from build123d import *

# Parameters (mm, degrees)
SKETCH1_R           = 1.95
SKETCH1_R_2         = 1.1
SKETCH1_R_3         = 1.7
SKETCH1_W           = 20
SKETCH1_H           = 3
BOSS_EXTRUDE2_DEPTH = 2


with BuildPart() as part:
    # Sketch1 → Boss-Extrude2 (new body)
    with BuildSketch(Plane.XY):
        with BuildLine():
            Line((-132.281780802, 145), (45.918219198, 145))
            ThreePointArc((45.918219198, 145), (47.332432761, 144.414213562), (47.918219198, 143))
            Line((47.918219198, 143), (47.918219198, 137))
            ThreePointArc((47.918219198, 137), (47.332432761, 135.585786438), (45.918219198, 135))
            Line((45.918219198, 135), (30.918219198, 135))
            ThreePointArc((30.918219198, 135), (30.211112417, 134.707106781), (29.918219198, 134))
            Line((29.918219198, 134), (29.918219198, 11))
            ThreePointArc((29.918219198, 11), (30.211112417, 10.292893219), (30.918219198, 10))
            Line((30.918219198, 10), (45.918219198, 10))
            ThreePointArc((45.918219198, 10), (47.332432761, 9.414213562), (47.918219198, 8))
            Line((47.918219198, 8), (47.918219198, 2))
            ThreePointArc((47.918219198, 2), (47.332432761, 0.585786438), (45.918219198, 0))
            Line((45.918219198, 0), (29.918219198, 0))
            Line((29.918219198, 0), (29.918219198, -44.1))
            ThreePointArc((29.918219198, -44.1), (29.62532598, -44.807106781), (28.918219198, -45.1))
            Line((28.918219198, -45.1), (4.418219198, -45.1))
            ThreePointArc((4.418219198, -45.1), (3.711112417, -44.807106781), (3.418219198, -44.1))
            Line((3.418219198, -44.1), (3.418219198, 0))
            Line((3.418219198, 0), (-4.181780802, 0))
            ThreePointArc((-4.181780802, 0), (-4.888887583, -0.292893219), (-5.181780802, -1))
            Line((-5.181780802, -1), (-5.181780802, -72))
            ThreePointArc((-5.181780802, -72), (-6.646246896, -75.535533906), (-10.181780802, -77))
            Line((-10.181780802, -77), (-18.181780802, -77))
            Line((-18.181780802, -77), (-18.181780802, -110))
            ThreePointArc((-18.181780802, -110), (-19.646246896, -113.535533906), (-23.181780802, -115))
            Line((-23.181780802, -115), (-63.181780802, -115))
            ThreePointArc((-63.181780802, -115), (-66.717314707, -113.535533906), (-68.181780802, -110))
            Line((-68.181780802, -110), (-68.181780802, -77))
            Line((-68.181780802, -77), (-76.181780802, -77))
            ThreePointArc((-76.181780802, -77), (-79.717314707, -75.535533906), (-81.181780802, -72))
            Line((-81.181780802, -72), (-81.181780802, -1))
            ThreePointArc((-81.181780802, -1), (-81.47467402, -0.292893219), (-82.181780802, 0))
            Line((-82.181780802, 0), (-89.781780802, 0))
            Line((-89.781780802, 0), (-89.781780802, -44.1))
            ThreePointArc((-89.781780802, -44.1), (-90.07467402, -44.807106781), (-90.781780802, -45.1))
            Line((-90.781780802, -45.1), (-115.281780802, -45.1))
            ThreePointArc((-115.281780802, -45.1), (-115.988887583, -44.807106781), (-116.281780802, -44.1))
            Line((-116.281780802, -44.1), (-116.281780802, 0))
            Line((-116.281780802, 0), (-132.281780802, 0))
            ThreePointArc((-132.281780802, 0), (-133.695994364, 0.585786438), (-134.281780802, 2))
            Line((-134.281780802, 2), (-134.281780802, 8))
            ThreePointArc((-134.281780802, 8), (-133.695994364, 9.414213562), (-132.281780802, 10))
            Line((-132.281780802, 10), (-117.281780802, 10))
            ThreePointArc((-117.281780802, 10), (-116.57467402, 10.292893219), (-116.281780802, 11))
            Line((-116.281780802, 11), (-116.281780802, 134))
            ThreePointArc((-116.281780802, 134), (-116.57467402, 134.707106781), (-117.281780802, 135))
            Line((-117.281780802, 135), (-132.281780802, 135))
            ThreePointArc((-132.281780802, 135), (-133.695994364, 135.585786438), (-134.281780802, 137))
            Line((-134.281780802, 137), (-134.281780802, 143))
            ThreePointArc((-134.281780802, 143), (-133.695994364, 144.414213562), (-132.281780802, 145))
        make_face()
        with Locations((-28.781780802, -111.2)):
            Circle(SKETCH1_R, mode=Mode.SUBTRACT)
        with Locations((41.918219198, 140)):
            Circle(SKETCH1_R_2, mode=Mode.SUBTRACT)
        with Locations((33.918219198, 140)):
            Circle(SKETCH1_R_2, mode=Mode.SUBTRACT)
        with Locations((41.918219198, 5)):
            Circle(SKETCH1_R_2, mode=Mode.SUBTRACT)
        with Locations((33.918219198, 5)):
            Circle(SKETCH1_R_2, mode=Mode.SUBTRACT)
        with Locations((-28.781780802, -83.8)):
            Circle(SKETCH1_R, mode=Mode.SUBTRACT)
        with Locations((-21.281780802, -62)):
            Circle(SKETCH1_R_3, mode=Mode.SUBTRACT)
        with Locations((-27.981780802, -33)):
            Circle(SKETCH1_R_3, mode=Mode.SUBTRACT)
        with Locations((-58.381780802, -33)):
            Circle(SKETCH1_R_3, mode=Mode.SUBTRACT)
        with Locations((-65.081780802, -62)):
            Circle(SKETCH1_R_3, mode=Mode.SUBTRACT)
        with Locations((-57.581780802, -83.8)):
            Circle(SKETCH1_R, mode=Mode.SUBTRACT)
        with Locations((-120.281780802, 5)):
            Circle(SKETCH1_R_2, mode=Mode.SUBTRACT)
        with Locations((-128.281780802, 5)):
            Circle(SKETCH1_R_2, mode=Mode.SUBTRACT)
        with Locations((-120.281780802, 140)):
            Circle(SKETCH1_R_2, mode=Mode.SUBTRACT)
        with Locations((-128.281780802, 140)):
            Circle(SKETCH1_R_2, mode=Mode.SUBTRACT)
        with Locations((-57.581780802, -111.2)):
            Circle(SKETCH1_R, mode=Mode.SUBTRACT)
        with Locations((-103.281780802, 140.5)):
            Rectangle(SKETCH1_W, SKETCH1_H, mode=Mode.SUBTRACT)
        with Locations((16.918219198, 140.5)):
            Rectangle(SKETCH1_W, SKETCH1_H, mode=Mode.SUBTRACT)
    extrude(amount=BOSS_EXTRUDE2_DEPTH)


solid = part.part
Check sheet for the modelled part. Datum: model origin and axes. Units: mm. Round coordinates to 2 decimals unless told otherwise and drop trailing zeros. Write each loop counter-clockwise with the first axis right and the second up, starting at its lowest first coordinate (ties: lowest second). Pieces come first, ordered by that corner, then holes. Notation, with made-up numbers: (20.5, 81.25) -> (53.5, 81.25) arc R19 cw to (53.5, 86.25) -> close; hole circle Ø9 at (-20.75, 67). An arc over 180 degrees is marked (long way). Answer as CSV lines item,"result". Start each with the question number.
1) Section check A-A on x = -110.5. Enter the section's corners in (y, z).
2) Section check C-C on x = -14. Enter the section's corners in (y, z), and give its area (3 significant figures).
3) Go/stop test with flat-tipped pins: P1, Ø1, axis at y = -30, z = 1, coming from the +X side; P2, Ø0.6, axis at x = -74, z = 0.5, coming from the -Y side; P3, Ø1, axis at x = 17, z = 1, coming from the -Y side; P4, Ø2.5, axis at x = -57.58, y = -111.2, coming from the -Z side. Record where each tip stops, or that it passes through.
4) Material ranges on line 1 (X direction, y = -8, z = 1.5); line 2 (Y direction, x = -125.5, z = 1.55); line 3 (X direction, y = -61.5, z = 1.65), recorded low to high. Write a range as from..to.
5) Section check D-D on y = 20. Enter the section's corners in (x, z).
6) Section check B-B on z = 1.4. State how many separate pieces and enclosed holes the cut face has, and give its area (3 significant figures).
Found:
1,outline,"(-45.1, 0) -> (139, 0) -> (139, 2) -> (-45.1, 2) -> close; (142, 0) -> (145, 0) -> (145, 2) -> (142, 2) -> close"
2,outline,"(-77, 0) -> (145, 0) -> (145, 2) -> (-77, 2) -> close"
2,area,"444 mm^2"
3,P1,"stops at x = 29.92"
3,P2,"stops at y = -77"
3,P3,"stops at y = -45.1"
3,P4,"passes through"
4,line 1,"x = -116.28..-89.78, -81.18..-5.18, 3.42..29.92"
4,line 2,"y = 0..10, 135..145"
4,line 3,"x = -81.18..-66.71, -63.46..-22.91, -19.66..-5.18"
5,outline,"(-116.28, 0) -> (29.92, 0) -> (29.92, 2) -> (-116.28, 2) -> close"
6,separate pieces,"1"
6,enclosed holes,"18"
6,area,"31,800 mm^2"
